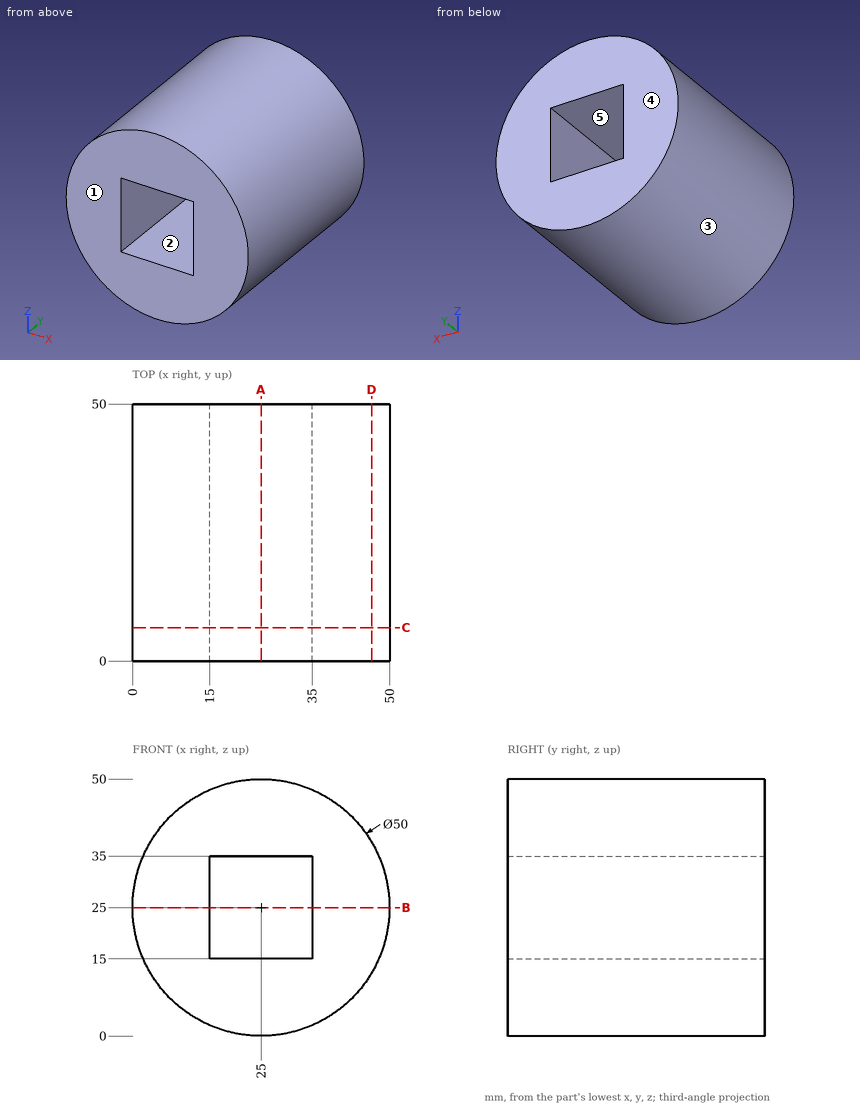
Verification items for this drawing (mm, ordinates from the low corner). A direction names the side the tool comes from. Round coordinates to 2 decimals unless told otherwise and drop trailing zeros. Loops run counter-clockwise (first coordinate to the right, second up) from the corner with the lowest first, then second, coordinate; pieces in that order, holes last. Notation, with made-up numbers: (63, 69.25) - (116, 69.25) arc R19 ccw to (116, 82.25) - close; hole circle Ø7 at (17.5, -20.75). An arc over 180 degrees is marked (long way). Answer as CSV lines item,"result". Start each with the question number.
Item 1: Release check for a two-part mould opening along Z. For the marked faces 1, 2 and 3 record: +Z half, -Z half, draft (parallel to the pull), parting line (faces both ways), or undercut.
Item 2: Section check B-B (z = 25). Record the boundary of the cut face in (x, y), and give its area (3 significant figures).
Item 3: Section check C-C (y = 6.5). Record the boundary of the cut face in (x, z).
Item 4: Section check D-D (x = 46.5). Record the boundary of the cut face in (y, z), and give its area (3 significant figures).
Item 5: Scan lines: line 1 (X direction, y = 30.5, z = 26); line 2 (X direction, y = 23, z = 34.5). Record each from-to range of solid material in increasing order. Write a range as [from, to].
Item 6: Section check A-A (x = 25). Record the boundary of the cut face in (y, z), and give its area (3 significant figures).
Item 7: Set-up check for the marked faces 4 and 5: record each of +Z, -Z, +X, -X, +Y, -Y from which the full face is reachable in a straight line by a thin tool's end or side.
Item 8: Depth check by flat-ended pin: P1, Ø6, axis at x = 26, y = 19, coming from the +Z side; P2, Ø10, axis at x = 31.5, y = 38.5, coming from the -Z side; P3, Ø6, axis at x = 10.5, y = 34.5, coming from the +Z side. Enter the tip coordinate at first touch or a pass-through.
Report:
1,face 1,"draft"
1,face 2,"undercut"
1,face 3,"parting line"
2,outline,"(0, 0) - (15, 0) - (15, 50) - (0, 50) - close; (35, 0) - (50, 0) - (50, 50) - (35, 50) - close"
2,area,"1,500 mm2"
3,outline,"circle Ø50 at (25, 25); hole (15, 15) - (35, 15) - (35, 35) - (15, 35) - close"
4,outline,"(0, 12.24) - (50, 12.24) - (50, 37.76) - (0, 37.76) - close"
4,area,"1,280 mm2"
5,line 1,"x = [0.02, 15], [35, 49.98]"
5,line 2,"x = [1.88, 15], [35, 48.12]"
6,outline,"(0, 0) - (50, 0) - (50, 15) - (0, 15) - close; (0, 35) - (50, 35) - (50, 50) - (0, 50) - close"
6,area,"1,500 mm2"
7,face 4,"+Z, -Z, +X, -X, +Y"
7,face 5,"+Y, -Y"
8,P1,"stops at z = 50"
8,P2,"stops at z = 0.05"
8,P3,"stops at z = 47.2"
